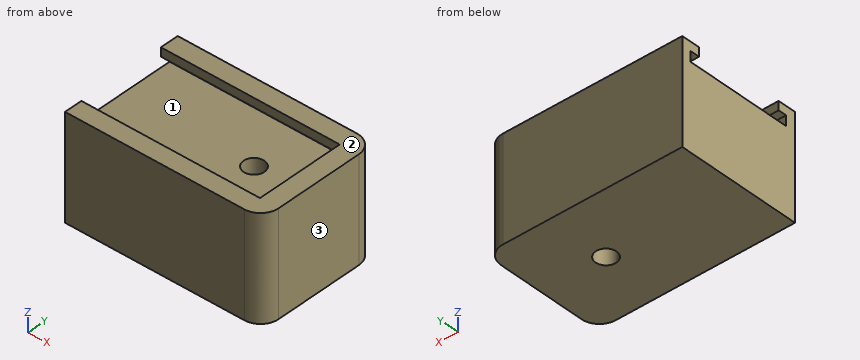
```python
from build123d import *

# Parameters (mm, degrees)
F0_W     = 38.1
F0_H     = 24.2
F1_DEPTH = 20
F2_W     = 34.5
F2_H     = 17.1
F3_DEPTH = 1.7
F4_W     = 34.6
F4_H     = 20.55
F5_DEPTH = 1.95
F6_R     = 3.5
F7_R     = 2
F8_DEPTH = 16.35


with BuildPart() as f1:
    # F0 (on Top) → F1 (new body)
    with BuildSketch(Plane.XY):
        with Locations((-19.05, 12.1)):
            Rectangle(F0_W, F0_H)
    extrude(amount=F1_DEPTH)

    # F2 (on face) → F3 (cut)
    with BuildSketch(Plane.XY.offset(20)):
        with Locations((-20.85, 12.05)):
            Rectangle(F2_W, F2_H)
    extrude(amount=-F3_DEPTH, mode=Mode.SUBTRACT)

    # F4 (on face) → F5 (cut)
    with BuildSketch(Plane.XY.offset(18.3)):
        with Locations((-20.8, 12.183178224)):
            Rectangle(F4_W, F4_H)
    extrude(amount=-F5_DEPTH, mode=Mode.SUBTRACT)

    # F6
    f6_edges = [f1.edges().sort_by_distance(p)[0] for p in [
        (0, 24.2, 10),
        (0, 0, 10),
    ]]
    fillet(f6_edges, radius=F6_R)

    # F7 (on face) → F8 (cut, through all)
    with BuildSketch(Plane.XY.offset(16.35)):
        with Locations((-12.5, 12.1)):
            Circle(F7_R)
    extrude(amount=-F8_DEPTH, mode=Mode.SUBTRACT)


solid = f1.part
```
The listing builds one solid part. Answer for the finished solid, in the listing's coordinates (mm). Face numbers are marked on the shaded views. Give positions to 0.01 mm unless a question says otherwise; leave off trailing zeros. Order: outer loops, then holes, each group sorted by start corner. A loop starts at its lowest first (then second) coordinate and runs counter-clockwise, first axis right, second up.
1) Consider line 1 along Y through (x, z) = (-12.5, 9.25); line 2 along Z through (x, y) = (-35, 2.25); line 3 along Z through (x, y) = (-21.5, 20.25). Determine where each line is inside the solid, lowest interval first.
Reported:
line 1: y = 0 to 10.1, 14.1 to 24.2
line 2: z = 0 to 16.35, 18.3 to 20
line 3: z = 0 to 16.35
2) Given P1, Ø1.9, axis at y = 13, z = 19, coming from the -X side; P2, Ø3, axis at x = -12.5, y = 12.1, coming from the +Z side; P3, Ø6, axis at x = -9.5, y = 15, coming from the -Z side; P4, Ø0.6, axis at y = 8, z = 17.5, coming from the -X side, each flat-ended and moving along its own axis, determine where each tip first touches the part or whether it passes through.
Reported:
P1: stops at x = -3.6
P2: passes through
P3: stops at z = 0
P4: stops at x = -3.5
3) Find section C-C on x = -12.5. Write down the section's boundary in (y, z).
Reported:
outline: (0, 0) - (10.1, 0) - (10.1, 16.35) - (1.91, 16.35) - (1.91, 18.3) - (3.5, 18.3) - (3.5, 20) - (0, 20) - close; (14.1, 0) - (24.2, 0) - (24.2, 20) - (20.6, 20) - (20.6, 18.3) - (22.46, 18.3) - (22.46, 16.35) - (14.1, 16.35) - close
4) Find section A-A on y = 12.1. Write down the section's boundary in (x, z), then the cut area to 3 significant figures.
Reported:
outline: (-38.1, 0) - (-14.5, 0) - (-14.5, 16.35) - (-38.1, 16.35) - close; (-10.5, 0) - (0, 0) - (0, 20) - (-3.6, 20) - (-3.6, 18.3) - (-3.5, 18.3) - (-3.5, 16.35) - (-10.5, 16.35) - close
area: 570 mm2
5) Find section D-D on y = 17. Write down the section's boundary in (x, z), then the cut area to 3 significant figures.
Reported:
outline: (-38.1, 0) - (0, 0) - (0, 20) - (-3.6, 20) - (-3.6, 18.3) - (-3.5, 18.3) - (-3.5, 16.35) - (-38.1, 16.35) - close
area: 636 mm2
6) Determine the mould class of the marked faces 1, 2 and 3 for opening direction Z: pulls with the +Z half, pulls with the -Z half, needs draft (parallel to the pull), parting line crosses it, or undercut.
Reported:
face 1: undercut
face 2: pulls with the +Z half
face 3: needs draft
7) Find section B-B on z = 11.75. Write down the section's boundary in (x, y).
Reported:
outline: (-38.1, 0) - (-3.5, 0) arc R3.5 ccw to (0, 3.5) - (0, 20.7) arc R3.5 ccw to (-3.5, 24.2) - (-38.1, 24.2) - close; hole circle Ø4 at (-12.5, 12.1)
